```python
from build123d import *

# Parameters (mm, degrees)
SKETCH_2_R          = 3.6
SKETCH_2_R_2        = 1.5
SKETCH_2_R_3        = 2
EXTRUDE_1_DEPTH     = 3
SKETCH_8_R          = 1
CUT_EXTRUDE_1_DEPTH = 105.27847333
FILLET_1_R          = 2
FILLET_2_R          = 6


with BuildPart() as part:
    # 草图2 → 凸台-拉伸1 (new body)
    with BuildSketch(Plane.XY):
        with BuildLine():
            Line((-65, 0), (-65, 44))
            Line((-65, 44), (-78.2, 61.6))
            ThreePointArc((-78.2, 61.6), (-77.728789328, 66.924672427), (-72.384272007, 67.026213321))
            Line((-72.384272007, 67.026213321), (-55, 52))
            Line((-55, 52), (-55, 44))
            Line((-55, 44), (-40, 44))
            Line((-40, 44), (-40, 19))
            Line((-40, 19), (-55, 19))
            Line((-55, 19), (-55, 4))
            Line((-55, 4), (-50, 4))
            Line((-50, 4), (-50, -5))
            Line((-50, -5), (-60, -5))
            ThreePointArc((-60, -5), (-63.535533906, -3.535533906), (-65, 0))
        make_face()
        with Locations((-60, 39)):
            Circle(SKETCH_2_R, mode=Mode.SUBTRACT)
        with Locations((-60, 0)):
            Circle(SKETCH_2_R, mode=Mode.SUBTRACT)
        with Locations((-75, 64)):
            Circle(SKETCH_2_R_2, mode=Mode.SUBTRACT)
        with Locations((-60, 19.75)):
            Circle(SKETCH_2_R_3, mode=Mode.SUBTRACT)
        with Locations((-60, 48)):
            Circle(SKETCH_2_R_3, mode=Mode.SUBTRACT)
        with Locations((-47.5, 37)):
            Circle(SKETCH_2_R_3, mode=Mode.SUBTRACT)
        with Locations((-47.5, 26)):
            Circle(SKETCH_2_R_3, mode=Mode.SUBTRACT)
    extrude(amount=EXTRUDE_1_DEPTH)

    # 草图8 → 切除-拉伸1 (cut, through all)
    with BuildSketch(Plane.XY.offset(3)):
        with Locations((-55, 45)):
            Circle(SKETCH_8_R)
        with Locations((-55, 18)):
            Circle(SKETCH_8_R)
        with Locations((-55, 5)):
            Circle(SKETCH_8_R)
    extrude(amount=-CUT_EXTRUDE_1_DEPTH, mode=Mode.SUBTRACT)

    # 圆角1
    fillet_1_edges = [part.edges().sort_by_distance(p)[0] for p in [
        (-55, 52, 1.5),
        (-40, 44, 1.5),
        (-40, 19, 1.5),
        (-65, 44, 1.5),
    ]]
    fillet(fillet_1_edges, radius=FILLET_1_R)

    # 圆角2
    fillet_2_edges = [part.edges().sort_by_distance(p)[0] for p in [
        (-50, -5, 1.5),
    ]]
    fillet(fillet_2_edges, radius=FILLET_2_R)


solid = part.part
```
Read the model definition and answer for the solid it produces. Units are mm, in the model's axes. A direction names the side the tool comes from. Give positions to 0.01 mm unless a question says otherwise; leave off trailing zeros. Write each loop counter-clockwise with the first axis right and the second up, starting at its lowest first coordinate (ties: lowest second). Pieces come first, ordered by that corner, then holes. Notation, with made-up numbers: (72.25, 6.25) - (76.25, 6.25) arc R14 ccw to (76.25, 16.25) - close; hole circle Ø8 at (-28, -40). An arc over 180 degrees is marked (long way). Write item = value, one per line. Start each with the question number.
Item 1: Find section A-A (x = -47.5). Give the vertices of the cut face in (y, z).
Item 2: Find section D-D (x = -75). Give the vertices of the cut face in (y, z).
Item 3: Find section B-B (y = 26). Give the vertices of the cut face in (x, z), then the cut area to 3 significant figures.
Item 4: Each of these flat-tipped pins is pushed along its axis until it touches: P1, Ø1.5, axis at y = 9, z = 1, coming from the +X side; P2, Ø1.5, axis at x = -53, z = 1, coming from the +Y side; P3, Ø1.5, axis at y = 57.5, z = 2, coming from the -X side. Where does it stop, or does it pass through?
Item 5: Find section C-C (z = 1.35). Give the vertices of the cut face in (x, y).
Item 6: Find the intervals of material crossed by probe 1 along Y at (x, z) = (-47.5, 2.7); probe 2 along Y at (x, z) = (-60, 1.8); probe 3 along X at (y, z) = (3, 2.25), in increasing order. Write a range as [from, to].
Item 7: The mould has two halves that part along X. Classify faces 1 (the cylindrical face through (-77.788, 66.868, 1.479)), 2 (the cylindrical face through (-59.077, 46.226, 1.479)), 3 (the flat face through (-64.155, 59.913, 1.479)), 4 (the cylindrical face through (-58.092, 20.351, 1.479)): +X half, -X half, draft (parallel to the pull), parting line (faces both ways), or undercut.
Item 8: A tool of negligible diameter and unlimited length cuts with its end or side. For faces 5 (the flat face through (-55, 12, 1)), 6 (the flat face through (-65, 21, 1)), 7 (the flat face through (-49, 44, 1)), from which of +Z, -Z, +X, -X, +Y, -Y can it reach the whole face along a straight path? Write none if from no direction.
Response:
q1.outline = (19, 0) - (24, 0) - (24, 3) - (19, 3) - close; (28, 0) - (35, 0) - (35, 3) - (28, 3) - close; (39, 0) - (44, 0) - (44, 3) - (39, 3) - close
q2.outline = (57.33, 0) - (62.5, 0) - (62.5, 3) - (57.33, 3) - close; (65.5, 0) - (68, 0) - (68, 3) - (65.5, 3) - close
q3.outline = (-65, 0) - (-49.5, 0) - (-49.5, 3) - (-65, 3) - close; (-45.5, 0) - (-40, 0) - (-40, 3) - (-45.5, 3) - close
q3.area = 63.0 mm²
q4.P1 = -55
q4.P2 = 44
q4.P3 = -75.69
q5.outline = (-78.2, 61.6) - (-65.4, 44.53) arc R2 cw to (-65, 43.33) - (-65, 0) arc R5 ccw to (-60, -5) - (-56, -5) arc R6 ccw to (-50, 1) - (-50, 4) - (-55, 4) arc R1 cw to (-55, 6) - (-55, 17) arc R1 cw to (-55, 19) - (-42, 19) arc R2 ccw to (-40, 21) - (-40, 42) arc R2 ccw to (-42, 44) - (-55, 44) arc R1 cw to (-55, 46) - (-55, 51.09) arc R2 ccw to (-55.69, 52.6) - (-72.38, 67.03) arc R4 ccw to start; hole circle Ø3 at (-75, 64); hole circle Ø7.2 at (-60, 0); hole circle Ø7.2 at (-60, 39); hole circle Ø4 at (-60, 19.75); hole circle Ø4 at (-60, 48); hole circle Ø4 at (-47.5, 26); hole circle Ø4 at (-47.5, 37)
q6.probe_1 = [19, 24], [28, 35], [39, 44]
q6.probe_2 = [-5, -3.6], [3.6, 17.75], [21.75, 35.4], [42.6, 46], [50, 56.32]
q6.probe_3 = [-65, -61.99], [-58.01, -50]
q7.face_1 = parting line
q7.face_2 = undercut
q7.face_3 = +X half
q7.face_4 = undercut
q8.face_5 = +Z, -Z, +X
q8.face_6 = +Z, -Z, -X, -Y
q8.face_7 = +Z, -Z, +X, +Y
